Answer from the drawing. Dimensions are ordinates in mm from the lowest x, y and z of the part. Give positions to 0.01 mm unless a question says otherwise; leave off trailing zeros. Loops run counter-clockwise (first coordinate to the right, second up) from the corner with the lowest first, then second, coordinate; pieces in that order, holes last.
Item 1: Section D-D, the plane z = 28 is taken. Give the vertices of the cut face in (x, y).
Item 2: Section A-A, the plane z = 82 is taken. Give the vertices of the cut face in (x, y), and give its area (3 significant figures).
Item 3: Section B-B, the plane y = 6 is taken. Give the vertices of the cut face in (x, z) (1 decimal).
Item 4: Section C-C, the plane x = 17 is taken. Give the vertices of the cut face in (y, z).
Item 5: Each of these flat-tipped pins is pushed along its axis until it touches: pin 1 Ø1 at (y, z) = (4.5, 24.5) entering from -X; pin 2 Ø3 at (x, y) = (234.5, 4) entering from -Z; pin 3 Ø5 at (x, y) = (54.5, 3.5) entering from -Z (1 decimal). Where does it stop, or does it pass through?
Item 6: Consider line 1 along Z through (x, y) = (199, 1); line 2 along Y through (x, z) = (251, 5.5); line 3 along Z through (x, y) = (49, 4.75) (1 decimal). Determine where each line is inside the solid, lowest interval first.
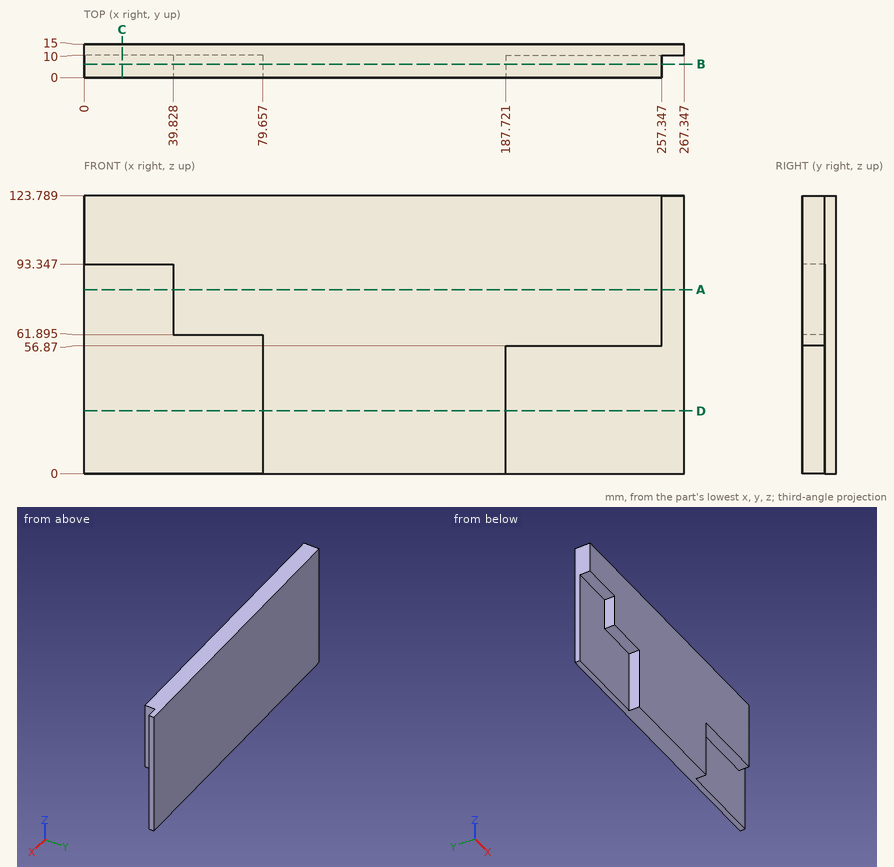
Worked answers:
1. outline: (0, 10) - (79.66, 10) - (79.66, 0) - (187.72, 0) - (187.72, 10) - (267.35, 10) - (267.35, 15) - (0, 15) - close
2. outline: (0, 10) - (39.83, 10) - (39.83, 0) - (257.35, 0) - (257.35, 10) - (267.35, 10) - (267.35, 15) - (0, 15) - close
2. area: 3,510 mm2
3. outline: (0, 93.3) - (39.8, 93.3) - (39.8, 61.9) - (79.7, 61.9) - (79.7, 0) - (187.7, 0) - (187.7, 56.9) - (257.3, 56.9) - (257.3, 123.8) - (0, 123.8) - close
4. outline: (0, 93.35) - (10, 93.35) - (10, 0) - (15, 0) - (15, 123.79) - (0, 123.79) - close
5. pin 1: stops at x = 79.66
5. pin 2: stops at z = 56.87
5. pin 3: stops at z = 61.9
6. line 1: z = 56.87 to 123.79
6. line 2: y = 10 to 15
6. line 3: z = 61.9 to 123.8
